Can you work these out from the model? Positions are in its coordinate system, mm. Face numbers are marked on the shaded views. A direction names the side the tool comes from. Give positions to 0.01 mm unless a question says otherwise; leave off trailing zeros. Order: outer loops, then holes, each group sorted by start corner. A loop starts at its lowest first (then second) coordinate and runs counter-clockwise, first axis right, second up. Notation, with made-up numbers: M 44.25,-9 L 80.25,-9 A22 cw 80.25,30 Z; hole C -2,9 d9. An arc over 180 degrees is marked long. Answer as a JSON object with one key per item and string values.
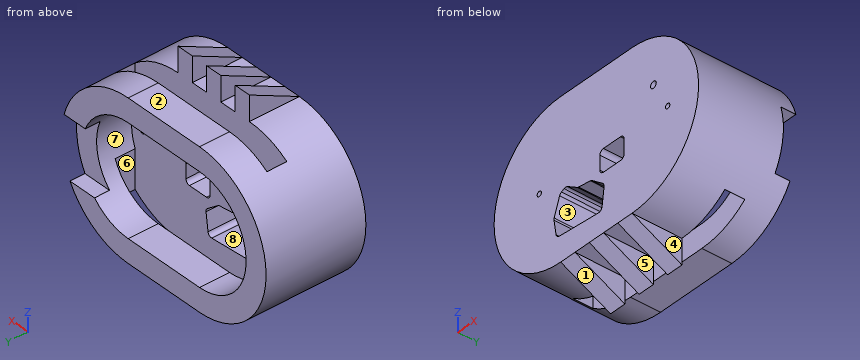
```python
from build123d import *

# Parameters (mm, degrees)
LIP_DEPTH                    = 6
BASE_DEPTH                   = 3
LAMDABREGMAGUIDES_DEPTH      = 5
LAMDABREGMAGUIDES_DEPTH_BACK = 5
SKETCH16_R                   = 0.15
SKETCH16_R_2                 = 0.2
SKETCH3_W                    = 10.638387248
SKETCH3_H                    = 1.2
CUT4ACRYLIC_DEPTH            = 10
SKETCH4_W                    = 2.35
SKETCH4_H                    = 3.533
CUTFORGROUNDPIN_DEPTH        = 0.9
BOSS_EXTRUDE6_DEPTH          = 1
CRVPATTERN1_START            = 3.5
CRVPATTERN1_DEPTH            = 1
CRVPATTERN1_START_2          = 5.5
CRVPATTERN1_2_DEPTH          = 1
BOSS_EXTRUDE7_DEPTH          = 1
CRVPATTERN5_START            = 3.5
CRVPATTERN5_DEPTH            = 1
CRVPATTERN5_START_2          = 5.5
CRVPATTERN5_2_DEPTH          = 1
CUT_EXTRUDE1_DEPTH           = 10
CUT_EXTRUDE3_DEPTH           = 10
CUT_EXTRUDE3_DEPTH_BACK      = 10
SKETCH32_W                   = 1.7
SKETCH32_H                   = 1.34
FILLET1_R                    = 0.25


# Read off the part's stored shape, not the designer's step: Lip, CrvPattern1, CrvPattern5
with BuildPart() as part:
    # Lip outline → Lip (new body)
    with BuildSketch(Plane(origin=(0, 0, 0), x_dir=(1, 0, 0), z_dir=(0, 1, 0))):
        with BuildLine():
            ThreePointArc((1.5, 4.6665), (-3.1665, 0), (1.5, -4.6665))
            Line((1.5, -4.6665), (6.5, -4.6665))
            ThreePointArc((6.5, -4.6665), (11.1665, 0), (6.5, 4.6665))
            Line((6.5, 4.6665), (1.5, 4.6665))
        make_face()
        with BuildLine():
            Line((6.5, -3.2665), (1.5, -3.2665))
            ThreePointArc((1.5, -3.2665), (-1.7665, 0), (1.5, 3.2665))
            Line((1.5, 3.2665), (6.5, 3.2665))
            ThreePointArc((6.5, 3.2665), (9.7665, 0), (6.5, -3.2665))
        make_face(mode=Mode.SUBTRACT)
    extrude(amount=LIP_DEPTH)

    # Sketch2 → Base (add)
    with BuildSketch(Plane(origin=(0, 0, 0), x_dir=(1, 0, 0), z_dir=(0, 1, 0))):
        with BuildLine():
            Line((6.5, -3.2665), (1.5, -3.2665))
            ThreePointArc((1.5, -3.2665), (-1.7665, 0), (1.5, 3.2665))
            Line((1.5, 3.2665), (6.5, 3.2665))
            ThreePointArc((6.5, 3.2665), (9.7665, 0), (6.5, -3.2665))
        make_face()
    extrude(amount=BASE_DEPTH)

    # Sketch16 → LamdaBregmaGuides (cut, two sides: drawn at the far end of the back side and taken through both)
    with BuildSketch(Plane(origin=(0, 0, 0), x_dir=(1, 0, 0), z_dir=(0, 1, 0)).offset(-LAMDABREGMAGUIDES_DEPTH_BACK)):
        with Locations(Location((0, 0, 0), (0, 0, 270))):
            Circle(SKETCH16_R)
        with Locations(Location((9, 0, 0), (0, 0, 270))):
            Circle(SKETCH16_R)
        with Locations(Location((8, -1.75, 0), (0, 0, 270))):
            Circle(SKETCH16_R_2)
    extrude(amount=LAMDABREGMAGUIDES_DEPTH + LAMDABREGMAGUIDES_DEPTH_BACK, mode=Mode.SUBTRACT)

    # Sketch3 → Cut4Acrylic (cut)
    with BuildSketch(Plane.XY.offset(4.6665)):
        with Locations((4.193105486, 3.6)):
            Rectangle(SKETCH3_W, SKETCH3_H)
    extrude(amount=-CUT4ACRYLIC_DEPTH, mode=Mode.SUBTRACT)

    # Sketch4 → CutforGroundPin (cut)
    with BuildSketch(Plane(origin=(0, 6, 0), x_dir=(1, 0, 0), z_dir=(0, 1, 0))):
        with Locations((10.030760676, 0.5)):
            Rectangle(SKETCH4_W, SKETCH4_H)
    extrude(amount=-CUTFORGROUNDPIN_DEPTH, mode=Mode.SUBTRACT)

    # Sketch21 → Boss-Extrude6 (add)
    with BuildSketch(Plane(origin=(1.5, 0, 0), x_dir=(0, 0, -1), z_dir=(1, 0, 0))):
        Polygon((-4.6665, 3), (-6.1665, 3), (-4.6665, 0), align=None)
    extrude(amount=BOSS_EXTRUDE6_DEPTH)

    # CrvPattern1 outline → CrvPattern1 (add)
    with BuildSketch(Plane.YZ.offset(CRVPATTERN1_START)):
        Polygon((0, 4.6665), (3, 4.6665), (3, 6.1665), align=None)
    extrude(amount=CRVPATTERN1_DEPTH)

    # CrvPattern1 2 outline → CrvPattern1 2 (add)
    with BuildSketch(Plane.YZ.offset(CRVPATTERN1_START_2)):
        Polygon((0, 4.6665), (3, 4.6665), (3, 6.1665), align=None)
    extrude(amount=CRVPATTERN1_2_DEPTH)

    # Sketch22 → Boss-Extrude7 (add)
    with BuildSketch(Plane(origin=(1.5, 0, 0), x_dir=(0, 0, -1), z_dir=(1, 0, 0))):
        Polygon((4.6665, 0), (4.6665, 3), (6.1665, 3), align=None)
    extrude(amount=BOSS_EXTRUDE7_DEPTH)

    # CrvPattern5 outline → CrvPattern5 (add)
    with BuildSketch(Plane.YZ.offset(CRVPATTERN5_START)):
        Polygon((0, -4.6665), (3, -6.1665), (3, -4.6665), align=None)
    extrude(amount=CRVPATTERN5_DEPTH)

    # CrvPattern5 2 outline → CrvPattern5 2 (add)
    with BuildSketch(Plane.YZ.offset(CRVPATTERN5_START_2)):
        Polygon((0, -4.6665), (3, -6.1665), (3, -4.6665), align=None)
    extrude(amount=CRVPATTERN5_2_DEPTH)

    # Sketch31 → Cut-Extrude1 (cut)
    with BuildSketch(Plane(origin=(0, 3, 0), x_dir=(1, 0, 0), z_dir=(0, 1, 0))):
        Polygon((1.21, 3.14), (1.02, 1.99), (1.46, 0.79), (1.86, 0.6), (2.7, 1.12), (3.65, 1.24), (4.56, 1.94), (4.37, 3.37), align=None)
    extrude(amount=-CUT_EXTRUDE1_DEPTH, mode=Mode.SUBTRACT)

    # Sketch32 → Cut-Extrude3 (cut, two sides: drawn at the far end of the back side and taken through both)
    with BuildSketch(Plane(origin=(0, 0, 0), x_dir=(1, 0, 0), z_dir=(0, 1, 0)).offset(-CUT_EXTRUDE3_DEPTH_BACK)):
        with Locations((5.1, 0.58)):
            Rectangle(SKETCH32_W, SKETCH32_H)
    extrude(amount=CUT_EXTRUDE3_DEPTH + CUT_EXTRUDE3_DEPTH_BACK, mode=Mode.SUBTRACT)

    # Fillet1
    fillet1_edges = [part.edges().sort_by_distance(p)[0] for p in [
        (1.21, 1.5, -3.14),
        (4.37, 1.5, -3.37),
        (4.56, 1.5, -1.94),
        (3.65, 1.5, -1.24),
        (2.7, 1.5, -1.12),
        (1.86, 1.5, -0.6),
        (1.46, 1.5, -0.79),
        (1.02, 1.5, -1.99),
        (5.95, 1.5, 0.09),
        (5.95, 1.5, -1.25),
        (4.25, 1.5, -1.25),
        (4.25, 1.5, 0.09),
    ]]
    fillet(fillet1_edges, radius=FILLET1_R)


solid = part.part
```
1) Thinking about a two-plate mould opening in Z: for the marked faces 1, 2 and 3, which applies, pulls with the +Z half, pulls with the -Z half, needs draft (parallel to the pull), parting line crosses it, or undercut?
Results found:
{"face 1": "pulls with the -Z half", "face 2": "pulls with the +Z half", "face 3": "undercut"}
2) For the marked faces 4, 5, 6, 7 and 8, which set-ups out of +Z, -Z, +X, -X, +Y, -Y let a thin tool reach every point of the face, with its end or its side?
Results found:
{"face 4": "-Z, +X, +Y, -Y", "face 5": "-Z, +Y, -Y", "face 6": "+Z, -Z", "face 7": "+Y", "face 8": "-Y"}
3) I want a section at A-A on x = 8. Write out the boundary of the cut face in (y, z).
Results found:
{"outline": "M 0,-4.42 L 3,-4.42 L 3,1.55 L 0,1.55 Z; M 0,1.95 L 3,1.95 L 3,4.42 L 0,4.42 Z; M 4.2,-4.42 L 6,-4.42 L 6,-2.9 L 4.2,-2.9 Z; M 4.2,2.9 L 6,2.9 L 6,4.42 L 4.2,4.42 Z"}
4) I want a section at D-D on y = 0.65. Count the separate pieces of the cut face and the enclosed holes in it, and give its area (3 significant figures).
Results found:
{"separate pieces": "1", "enclosed holes": "5", "area": "107 mm²"}
5) I want a section at B-B on z = 1.75. Write out the boundary of the cut face in (x, y).
Results found:
{"outline": "M -2.83,0 L 7.8,0 L 7.8,3 L -1.26,3 L -1.26,6 L -2.83,6 Z; M 8.2,0 L 10.83,0 L 10.83,6 L 9.26,6 L 9.26,4.2 L 9.51,4.2 L 9.51,3 L 8.2,3 Z"}
6) I want a section at C-C on z = -5. Write out the boundary of the cut face in (x, y).
Results found:
{"outline": "M 1.5,0.67 L 2.5,0.67 L 2.5,3 L 1.5,3 Z; M 3.5,0.67 L 4.5,0.67 L 4.5,3 L 3.5,3 Z; M 5.5,0.67 L 6.5,0.67 L 6.5,3 L 5.5,3 Z"}
7) I'm going to push flat-ended pins straight in: pin 1 Ø0.8 at (x, y) = (3, 1) entering from +Z; pin 2 Ø0.9 at (x, y) = (4.5, 5.5) entering from -Z; pin 3 Ø1 at (x, y) = (10, 6) entering from +Z. Where does each tip first touch, or does it pass through?
Results found:
{"pin 1": "stops at z = 4.67", "pin 2": "stops at z = -4.67", "pin 3": "stops at z = 3.57"}
8) I need wall thicknesses on L1, parallel to X at y = 1.8, z = 0; L2, parallel to Z at x = 5.5, y = 4.9; L3, parallel to Y at x = 3.5, z = -3.75. Which ranges of each line are inside material? Lowest first, please.
Results found:
{"L1": "x = -3.17 to -0.15, 0.15 to 4.31, 5.89 to 8.85, 9.15 to 11.17", "L2": "z = -4.67 to -3.27, 3.27 to 4.67", "L3": "y = 0 to 3, 4.2 to 6"}
